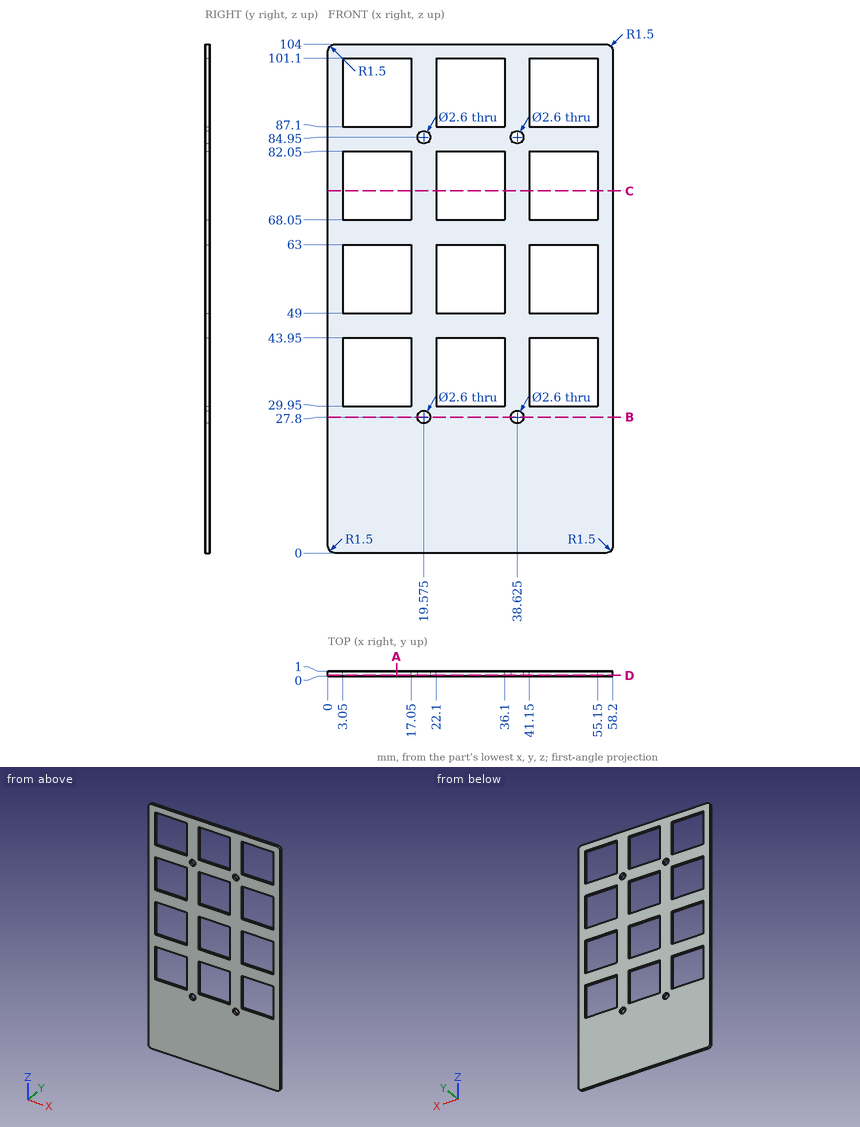
Design review of the part shown in the three views and the two pictorial views. Dimensions are in mm from the part's minimum x, y and z. Coordinates: 2 decimals unless noted, no trailing zeros. Loops run counter-clockwise (first coordinate to the right, second up) from the corner with the lowest first, then second, coordinate; pieces in that order, holes last. Notation, with made-up numbers: (19, 60) -> (60, 60) arc R16 ccw to (60, 78) -> close; hole circle Ø5 at (45.25, -11.75). An arc over 180 degrees is marked (long way). Answer as CSV lines item,"result".
Item 1: For L1, parallel to X at y = 0.6, z = 27.8 (3 decimals); L2, parallel to Z at x = 30, y = 0.5; L3, parallel to X at y = 0.8, z = 41, list the stretches that pass through material, from the lowest coordinate up.
Results below:
L1,"x = 0 to 18.275, 20.875 to 37.325, 39.925 to 58.2"
L2,"z = 0 to 29.95, 43.95 to 49, 63 to 68.05, 82.05 to 87.1, 101.1 to 104"
L3,"x = 0 to 3.05, 17.05 to 22.1, 36.1 to 41.15, 55.15 to 58.2"
Item 2: Take a section at A-A, the plane x = 14. State the section outline as (y, z) points, and give its area (3 significant figures).
Results below:
outline,"(0, 0) -> (1, 0) -> (1, 29.95) -> (0, 29.95) -> close; (0, 43.95) -> (1, 43.95) -> (1, 49) -> (0, 49) -> close; (0, 63) -> (1, 63) -> (1, 68.05) -> (0, 68.05) -> close; (0, 82.05) -> (1, 82.05) -> (1, 87.1) -> (0, 87.1) -> close; (0, 101.1) -> (1, 101.1) -> (1, 104) -> (0, 104) -> close"
area,"48.0 mm2"
Item 3: Take a section at C-C, the plane z = 74. State the section outline as (x, y) points, and give its area (3 significant figures).
Results below:
outline,"(0, 0) -> (3.05, 0) -> (3.05, 1) -> (0, 1) -> close; (17.05, 0) -> (22.1, 0) -> (22.1, 1) -> (17.05, 1) -> close; (36.1, 0) -> (41.15, 0) -> (41.15, 1) -> (36.1, 1) -> close; (55.15, 0) -> (58.2, 0) -> (58.2, 1) -> (55.15, 1) -> close"
area,"16.2 mm2"
Item 4: Take a section at D-D, the plane y = 0.15. Count the separate pieces of the cut face and the enclosed holes in it, and give its area (3 significant figures).
Results below:
separate pieces,"1"
enclosed holes,"16"
area,"3,680 mm2"
Item 5: Take a section at B-B, the plane z = 27.8. State the section outline as (x, y) points (3 decimals), and give its area (3 significant figures).
Results below:
outline,"(0, 0) -> (18.275, 0) -> (18.275, 1) -> (0, 1) -> close; (20.875, 0) -> (37.325, 0) -> (37.325, 1) -> (20.875, 1) -> close; (39.925, 0) -> (58.2, 0) -> (58.2, 1) -> (39.925, 1) -> close"
area,"53.0 mm2"
